Model file for the job. Use its own axes, mm. Coordinates: 2 decimals unless noted, no trailing zeros. Order: outer loops, then holes, each group sorted by start corner. A loop starts at its lowest first (then second) coordinate and runs counter-clockwise, first axis right, second up. Notation, with made-up numbers: M 7.5,86.25 L 32.5,86.25 A10 cw 32.5,92.25 Z; hole C 80.25,89.5 d3. An arc over 180 degrees is marked long. Return JSON: item names as keys, results as strings.
```python
from build123d import *

# Parameters (mm, degrees)
BOSS_EXTRUDE2_DEPTH = 2743.2
CUT_EXTRUDE1_DEPTH  = 128


with BuildPart() as part:
    # Sketch3 → Boss-Extrude2 (new body)
    with BuildSketch(Plane(origin=(0, 0, 0), x_dir=(1, 0, 0), z_dir=(0, 1, 0))):
        Polygon((0, 0), (43.18, 0), (43.18, 7.62), (5.330413857, 7.62), (5.330413857, 119.38), (43.18, 119.38), (43.18, 127), (0, 127), align=None)
    extrude(amount=BOSS_EXTRUDE2_DEPTH)

    # Sketch5 → Cut-Extrude1 (cut, through all)
    with BuildSketch(Plane.XY):
        Polygon((0, 2743.2), (43.18, 2700.02), (43.18, 2743.2), align=None)
    extrude(amount=-CUT_EXTRUDE1_DEPTH, mode=Mode.SUBTRACT)


solid = part.part
```
Item 1: Drop flat-ended pins along their axis: pin 1 Ø3 at (y, z) = (1573, -57.5) entering from +X; pin 2 Ø10 at (x, z) = (9.5, -24.5) entering from +Y. Give the stop position or say it passes through.
Check result:
{"pin 1": "stops at x = 5.33", "pin 2": "stops at y = 2738.7"}
Item 2: Saw through at C-C (z = -27). Write the cut outline in (x, y).
Check result:
{"outline": "M 0,0 L 5.33,0 L 5.33,2737.87 L 0,2743.2 Z"}
Item 3: Saw through at A-A (x = 27.5). Write the cut outline in (y, z).
Check result:
{"outline": "M 0,-127 L 2715.7,-127 L 2715.7,-119.38 L 0,-119.38 Z; M 0,-7.62 L 2715.7,-7.62 L 2715.7,0 L 0,0 Z"}
Item 4: Wall check: line 1 (Z direction, x = 26, y = 773); line 2 (X direction, y = 1555.5, z = -104.5); line 3 (Y direction, x = 4, z = -14.5). Give the ranges that are in metal, low to high.
Check result:
{"line 1": "z = -127 to -119.38, -7.62 to 0", "line 2": "x = 0 to 5.33", "line 3": "y = 0 to 2739.2"}
Item 5: Pull direction Z, two halves, no side cores. Call faces 1 (the flat face through (22, 1352, -127)), 2 (the flat face through (5.33, 1350, -63)), 3 (the flat face through (4, 0, -64)): +Z half, -Z half, draft (parallel to the pull), parting line (faces both ways), or undercut.
Check result:
{"face 1": "-Z half", "face 2": "undercut", "face 3": "draft"}
Item 6: Saw through at B-B (y = 343). Write the cut outline in (x, z), and give its area (3 significant figures).
Check result:
{"outline": "M 0,-127 L 43.18,-127 L 43.18,-119.38 L 5.33,-119.38 L 5.33,-7.62 L 43.18,-7.62 L 43.18,0 L 0,0 Z", "area": "1,250 mm2"}
